Autodesk Inventor part; units mm, degrees
ref_plane "YZ Plane" through (0, 0, 0) normal (1, 0, 0) x (0, 1, 0)
ref_plane "XZ Plane" through (0, 0, 0) normal (0, 1, 0) x (-1, 0, 0)
ref_plane "XY Plane" through (0, 0, 0) normal (0, 0, 1) x (1, 0, 0)
sketch "Sketch1" plane through (0, 0, 0) normal (0, 0, 1) x (1, 0, 0)
  line L0 (0, 13.97) -> (0, 0)
  line L1 (0, 0) -> (24.8666, 0)
  line L2 (24.8666, 0) -> (24.8666, 13.97)
  line L3 (23.5966, 13.97) -> (23.5966, 1.27)
  line L4 (23.5966, 1.27) -> (1.27, 1.27)
  line L5 (1.27, 1.27) -> (1.27, 13.97)
  line L6 (24.8666, 13.97) -> (23.5966, 13.97)
  line L7 (1.27, 13.97) -> (0, 13.97)
  dimension "d0" = 24.8666
  dimension "d2" = 13.97
  dimension "d3" = 1.27
  dimension "d4" = 1.27
  dimension "d5" = 1.27
extrude "Extrusion1" add sketch "Sketch1" along normal blind 355.6
sketch "Sketch2" plane through (24.8666, 0, 0) normal (1, 0, 0) x (0, 0, -1)
  line L0 (0, 13.97) -> (0, 0)
  line L1 (-355.6, 0) -> (-355.6, 13.97)
  circle A0 centre (-342.9, 6.985) radius 4.0005
  circle A1 centre (-12.7, 6.985) radius 4.0005
  dimension "d8" = 8.001
  dimension "d9" = 8.001
  dimension "d10" = 12.7
  dimension "d11" = 12.7
extrude "Extrusion2" cut sketch "Sketch2" against normal blind 317.5 contours A1
sketch "Sketch3" plane through (24.8666, 0, 0) normal (1, 0, 0) x (0, 0, -1)
  line L0 (-355.6, 0) -> (-355.6, 13.97)
  circle A0 centre (-342.9, 6.985) radius 4.0005
  dimension "d14" = 8.001
  dimension "d15" = 12.7
extrude "Extrusion3" cut sketch "Sketch3" against normal blind 317.5
properties part number "U-Channel"
Geometry check sheet. Reference: the model listing, model coordinates, mm. A direction names the side the tool comes from. Give positions to 0.01 mm unless a question says otherwise; leave off trailing zeros. Write each loop counter-clockwise with the first axis right and the second up, starting at its lowest first coordinate (ties: lowest second). Pieces come first, ordered by that corner, then holes. Notation, with made-up numbers: M 15,5 L 30,5 A19 ccw 30,31 Z; hole C 20,-8 d9. An arc over 180 degrees is marked long. One line per question, with ' | ' between items.
1. Mould release check, pull along Z, two halves, no side actions. Record for faces 1 (the face through (12, 1, 355.6)), 2 (the face through (0, 7, 175)), 3 (the face through (0.644, 8.187, 339.084)), 4 (the face through (12, 1, 0)): released by +Z, released by -Z, zero draft, split by the parting line, or undercut.
Ans:
face 1: released by +Z | face 2: zero draft | face 3: undercut | face 4: released by -Z
2. Cross-section at B-B (z = 144). Enter the section's corners in (x, y).
Ans:
outline: M 0,0 L 24.87,0 L 24.87,13.97 L 23.6,13.97 L 23.6,1.27 L 1.27,1.27 L 1.27,13.97 L 0,13.97 Z
3. Gauge pin test, flat ends, axial feed: pin 1 (3 mm diameter, centred on x = 19, y = 3.5, fed in from +Z); pin 2 (5 mm diameter, centred on x = 4.5, z = 305.5, fed in from +Y); pin 3 (10 mm diameter, centred on x = 3.5, z = 199, fed in from +Y). Record the tip position at first contact, or that the pin passes through.
Ans:
pin 1: through | pin 2: y = 1.27 | pin 3: y = 13.97
4. Set-up check for faces 5 (the face through (24.24, 5.453, 9.005)), 6 (the face through (13, 1.27, 175)): record each of +Z, -Z, +X, -X, +Y, -Y from which the full face is reachable in a straight line by a thin tool's end or side.
Ans:
face 5: +X, -X | face 6: +Z, -Z, +Y
5. Scan lines: line 1 along X through (y, z) = (9, 31); line 2 along Y through (x, z) = (24, 342.9); line 3 along Y through (x, z) = (2, 91). Record each from-to range of solid material in increasing order. Write a range as from..to.
Ans:
line 1: 0..1.27, 23.6..24.87 | line 2: 0..2.98, 10.99..13.97 | line 3: 0..1.27
6. Cross-section at A-A (z = 12.7). Enter the section's corners in (x, y), plus the area to 3 significant figures.
Ans:
outline: M 0,0 L 24.87,0 L 24.87,2.98 L 23.6,2.98 L 23.6,1.27 L 1.27,1.27 L 1.27,2.98 L 0,2.98 Z; M 0,10.99 L 1.27,10.99 L 1.27,13.97 L 0,13.97 Z; M 23.6,10.99 L 24.87,10.99 L 24.87,13.97 L 23.6,13.97 Z | area: 43.5 mm2
7. Cross-section at C-C (x = 18.25). Enter the section's corners in (y, z).
Ans:
outline: M 0,0 L 1.27,0 L 1.27,355.6 L 0,355.6 Z
